Autodesk Inventor part; units mm, degrees
ref_plane "Work Plane1" through (5, 0, 0) normal (1, 0, 0) x (0, 0, -1)
ref_plane "Work Plane2" through (5, -8.65, 23.4559) normal (0, 1, 0) x (1, 0, 0)
ref_plane "YZ Plane" through (0, 0, 0) normal (1, 0, 0) x (0, 1, 0)
sketch "Sketch1" plane through (0, 0, 0) normal (1, 0, 0) x (0, 1, 0)
  circle A0 centre (0, 0) radius 22.5
  circle A1 centre (0, 0) radius 40
  circle A2 centre (0, 36.75) radius 1.5
  circle A3 centre (0, 25.5) radius 1.5
  line L0 (0, 22.5) -> (0, 25.5)
  circle A4 centre (-36.75, 0) radius 1.5
  circle A5 centre (-25.5, 0) radius 1.5
  circle A6 centre (0, -36.75) radius 1.5
  circle A7 centre (0, -25.5) radius 1.5
  circle A8 centre (36.75, 0) radius 1.5
  circle A9 centre (25.5, 0) radius 1.5
  dimension "d0" = 45
  dimension "d9" = 80
  dimension "d12" = 3
  dimension "d13" = 3
  dimension "d64" = 3
  dimension "d67" = 360
ref_plane "Work Plane1" through (5, 0, 0) normal (1, 0, 0) x (0, 0, -1)
sketch "Sketch2" plane through (5, 0, 0) normal (1, 0, 0) x (0, 0, -1)
  line L0 (0, 0) -> (0, -8.65)
  line L1 (0, -8.65) -> (23.4559, -8.65)
  line L2 (0, -8.65) -> (-23.4559, -8.65)
  line L3 (-23.4559, -8.65) -> (-30.4559, -8.65)
  line L4 (23.4559, -8.65) -> (30.4559, -8.65)
  line L5 (-30.4559, -8.65) -> (-30.4559, -13.65)
  line L6 (-30.4559, -13.65) -> (30.4559, -13.65)
  line L7 (30.4559, -13.65) -> (30.4559, -8.65)
  circle A0 centre (0, 0) radius 22.5
  dimension "d20" = 8.65
  dimension "d21" = 7
  dimension "d22" = 7
  dimension "d23" = 5
  dimension "d50" = 45
extrude "Extrusion2" add sketch "Sketch2" against normal blind 45 contours L1 A0 L6 L2 | L1 L4 L7 L6 A0 | A0 L6 L5 L3 L2
ref_plane "Work Plane2" through (5, -8.65, 23.4559) normal (0, 1, 0) x (1, 0, 0)
sketch "Sketch3" plane through (5, -8.65, 23.4559) normal (0, 1, 0) x (1, 0, 0)
  line L0 (-5, 23.4559) -> (-8.8, 23.4559)
  circle A0 centre (-8.8, 35.9559) radius 1.5
  circle A1 centre (-38.3, 35.9559) radius 1.5
  line L1 (-45, 53.9117) -> (-45, -7)
  circle A2 centre (-22.8, -1.9441) radius 2.5527
  circle A3 centre (-22.8, 48.8559) radius 2.5527
  line L2 (-8.8, 35.9559) -> (-38.3, 35.9559)
  line L3 (-8.8, 23.4559) -> (-8.8, 35.9559)
  line L4 (-8.8, 35.9559) -> (-8.8, 23.4559)
  circle A4 centre (-8.8, 10.9559) radius 1.5
  circle A5 centre (-38.3, 10.9559) radius 1.5
  line L5 (-8.8, 10.9559) -> (-38.3, 10.9559)
  line L6 (-8.8, 23.4559) -> (-8.8, 10.9559)
  dimension "d26" = 3.8
  dimension "d31" = 3
  dimension "d32" = 3
  dimension "d39" = 5.1054
  dimension "d40" = 5.1054
  dimension "d57" = 29.5
  dimension "d61" = 12.5
extrude "Extrusion3" cut sketch "Sketch3" against normal blind 50
extrude "Extrusion4" add sketch "Sketch1" along normal blind 5 contours A1 | A4 | A5 | A6 | A7 | A8 | A9
sketch "Sketch4" plane through (5, 0, 0) normal (1, 0, 0) x (0, 0, -1)
  circle A0 centre (0, 0) radius 40
  circle A1 centre (0, 0) radius 27
  line L0 (0, 0) -> (-31.9454, 24.0726)
  line L1 (-35, 0) -> (0, 0)
  line L2 (0, 0) -> (0, 35)
  line L3 (0, 0) -> (-24.0726, 31.9454)
  arc A2 (-16.249, 21.5632) -> (-21.5632, 16.249) centre (0, 0) ccw
  dimension "d51" = 54
  dimension "d53" = 37
  dimension "d54" = 37
extrude "Extrusion5" cut sketch "Sketch4" against normal blind 24.5 contours L3 A1 L0 A0 picked at (-25.4889, 24.8968)
fillet "Fillet1" radius 2 10 edges at (2.5, 31.9454, 24.0726) (2.5, 24.0726, 31.9454) (2.5, 16.249, 21.5632) (2.5, 21.5632, 16.249) (-40, -11.15, 30.4559) (-40, -11.15, -30.4559) (2.5, -8.65, -20.7708) (2.5, -8.65, 20.7708) (2.5, -13.65, 17.8865) (2.5, -13.65, -17.8865)
extrude "Extrusion6" cut sketch "Sketch1" along normal blind 24.5 contours A4 | A5 | A6 | A7 | A8 | A9
properties part number "JeVois Camera Mount"
Geometry check sheet. Reference: the model listing, model coordinates, mm. A direction names the side the tool comes from. Coordinates: 2 decimals unless noted, no trailing zeros. Order: outer loops, then holes, each group sorted by start corner. A loop starts at its lowest first (then second) coordinate and runs counter-clockwise, first axis right, second up.
Q1. Draft check along Z on faces 1 (the face through (0, 17, -17)), 2 (the face through (2.465, 21.713, 17.017)), 3 (the face through (-19, -11, 30.456)). Enter one of: released by +Z, released by -Z, zero draft, split by the parting line, or undercut.
Reply:
face 1: zero draft
face 2: undercut
face 3: released by +Z
Q2. Sectioned sample at D-D on z = 4. Record the cut outline in (x, y), and give its area (3 significant figures).
Reply:
outline: (-40, -13.65) - (5, -13.65) - (5, -8.65) - (-40, -8.65) - close; (0, -39.8) - (5, -39.8) - (5, -22.14) - (0, -22.14) - close; (0, 22.14) - (5, 22.14) - (5, 39.8) - (0, 39.8) - close
area: 402 mm2
Q3. Tool access check on faces 4 (the face through (2.46, 17.02, 21.67)), 5 (the face through (-19, -11, -30.456)), 6 (the face through (2.5, 23.2, 31.9)). Record the directions out of +Z, -Z, +X, -X, +Y, -Y that give a thin tool (end or side, any length) a straight path to the whole face; none if there is none.
Reply:
face 4: +X, -X
face 5: -Z, -X, +Y, -Y
face 6: +X, -X, +Y
Q4. Sectioned sample at C-C on y = 25.5. Record the cut outline in (x, z), and give its area (3 significant figures).
Reply:
outline: (0, -30.82) - (5, -30.82) - (5, -1.5) - (0, -1.5) - close; (0, 1.5) - (5, 1.5) - (5, 19.22) - (0, 19.22) - close
area: 235 mm2
Q5. Depth check by flat-ended pin: pin 1 Ø3 at (x, y) = (-4, -8) entering from +Z; pin 2 Ø2 at (y, z) = (4, -22) entering from -X; pin 3 Ø6 at (x, z) = (-5, -25) entering from +Y. Enter the tip coordinate at first touch or a pass-through.
Reply:
pin 1: stops at z = 30.46
pin 2: stops at x = 0
pin 3: stops at y = -8.65
Q6. Thickness scan on probe 1 along Z at (x, y) = (-3.8, -12.4); probe 2 along X at (y, z) = (-12, 12.5); probe 3 along X at (y, z) = (-11.8, -25.4). Record the ranges inside material, lowest first.
Reply:
probe 1: z = -30.46 to -14, -11 to 11, 14 to 30.46
probe 2: x = -40 to -34.8, -31.8 to -5.3, -2.3 to 5
probe 3: x = -40 to -20.35, -15.25 to 5
Q7. Sectioned sample at A-A on x = -3.8. Record the cut outline in (y, z).
Reply:
outline: (-13.65, -30.46) - (-8.65, -30.46) - (-8.65, -14) - (-13.65, -14) - close; (-13.65, -11) - (-8.65, -11) - (-8.65, 11) - (-13.65, 11) - close; (-13.65, 14) - (-8.65, 14) - (-8.65, 30.46) - (-13.65, 30.46) - close
Q8. Sectioned sample at B-B on y = 0. Record the cut outline in (x, z), and give its area (3 significant figures).
Reply:
outline: (0, -40) - (5, -40) - (5, -38.25) - (0, -38.25) - close; (0, -35.25) - (5, -35.25) - (5, -27) - (0, -27) - close; (0, -24) - (5, -24) - (5, -22.5) - (0, -22.5) - close; (0, 22.5) - (5, 22.5) - (5, 24) - (0, 24) - close; (0, 27) - (5, 27) - (5, 35.25) - (0, 35.25) - close; (0, 38.25) - (5, 38.25) - (5, 40) - (0, 40) - close
area: 115 mm2
